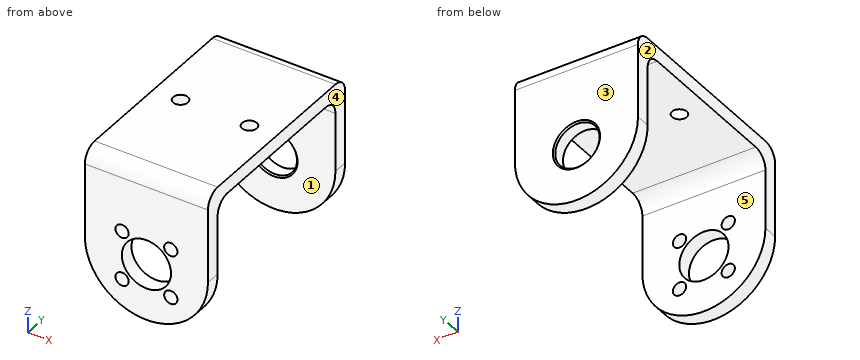
from build123d import *

# Parameters (mm, degrees)
BOSS_EXTRUDE3_DEPTH = 21.25
SHELL1_T            = -3
SKETCH6_R           = 4.5
CUT_EXTRUDE4_DEPTH  = 8.5
SKETCH8_R           = 1.347336496
CUT_EXTRUDE5_DEPTH  = 6
SKETCH9_R           = 1.5
CUT_EXTRUDE6_DEPTH  = 10
FILLET1_R           = 3
SKETCH11_R          = 5
CUT_EXTRUDE7_DEPTH  = 10
CHAMFER1_SIZE       = 0.3


with BuildPart() as part:
    # Sketch3 → Boss-Extrude3 (new, symmetric)
    with BuildSketch(Plane(origin=(0, 0, 0), x_dir=(1, 0, 0), z_dir=(0, 1, 0))):
        with BuildLine():
            Line((-12.5, 4), (12.5, 4))
            Line((12.5, 4), (12.5, 22))
            ThreePointArc((12.5, 22), (0, 34.5), (-12.5, 22))
            Line((-12.5, 22), (-12.5, 4))
        make_face()
    extrude(amount=BOSS_EXTRUDE3_DEPTH, both=True)

    # Shell1
    shell1_openings = [part.faces().sort_by_distance(p)[0] for p in [
        (0, 0, -34.5),
        (12.5, 0, -13),
        (-12.5, 0, -13),
    ]]
    offset(amount=SHELL1_T, openings=shell1_openings, kind=Kind.INTERSECTION)

    # Sketch6 → Cut-Extrude4 (cut)
    with BuildSketch(Plane(origin=(0, 21.25, 0), x_dir=(1, 0, 0), z_dir=(0, 1, 0))):
        with Locations(Location((0, 23, 0), (0, 0, 270))):
            Circle(SKETCH6_R)
    extrude(amount=-CUT_EXTRUDE4_DEPTH, mode=Mode.SUBTRACT)

    # Sketch8 → Cut-Extrude5 (cut)
    with BuildSketch(Plane(origin=(0, -21.25, 0), x_dir=(-1, 0, 0), z_dir=(0, -1, 0))):
        with Locations(Location((4.949747468, 18.050252532, 0), (0, 0, 90))):
            Circle(SKETCH8_R)
        with Locations(Location((-4.949747468, 18.050252532, 0), (0, 0, 90))):
            Circle(SKETCH8_R)
        with Locations(Location((-4.949747468, 27.949747468, 0), (0, 0, 90))):
            Circle(SKETCH8_R)
        with Locations(Location((4.949747468, 27.949747468, 0), (0, 0, 90))):
            Circle(SKETCH8_R)
    extrude(amount=-CUT_EXTRUDE5_DEPTH, mode=Mode.SUBTRACT)

    # Sketch9 → Cut-Extrude6 (cut)
    with BuildSketch(Plane(origin=(0, 0, -7), x_dir=(-1, 0, 0), z_dir=(0, 0, -1))):
        with Locations((-7, 0)):
            Circle(SKETCH9_R)
        with Locations((7, 0)):
            Circle(SKETCH9_R)
    extrude(amount=-CUT_EXTRUDE6_DEPTH, mode=Mode.SUBTRACT)

    # Fillet1
    fillet1_edges = [part.edges().sort_by_distance(p)[0] for p in [
        (0, -18.25, -7),
        (0, 18.25, -7),
        (0, -21.25, -4),
        (0, 21.25, -4),
    ]]
    fillet(fillet1_edges, radius=FILLET1_R)

    # Sketch11 → Cut-Extrude7 (cut)
    with BuildSketch(Plane(origin=(0, -18.25, 0), x_dir=(1, 0, 0), z_dir=(0, 1, 0))):
        with Locations(Location((0, 23, 0), (0, 0, 270))):
            Circle(SKETCH11_R)
    extrude(amount=-CUT_EXTRUDE7_DEPTH, mode=Mode.SUBTRACT)

    # Chamfer1
    chamfer1_edges = [part.edges().sort_by_distance(p)[0] for p in [
        (0, 18.25, -27.5),
        (0, 21.25, -27.5),
    ]]
    chamfer(chamfer1_edges, length=CHAMFER1_SIZE)


solid = part.part
Source: CAD feature listing. Evaluate the final solid. Frame: model axes, mm. Face numbers are marked on the shaded views. A direction names the side the tool comes from. Coordinates: 2 decimals unless noted, no trailing zeros. Loops run counter-clockwise (first coordinate to the right, second up) from the corner with the lowest first, then second, coordinate; pieces in that order, holes last. Notation, with made-up numbers: (34.25, 67.5) -> (72.25, 67.5) arc R31 ccw to (72.25, 99.5) -> close; hole circle Ø10 at (82.5, 87). An arc over 180 degrees is marked (long way). Answer in a Markdown table with one row per item. Add a question column.
Q1. Section D-D on z = -30.5. Return the cut outline in (x, y), and give its area (3 significant figures).
Q2. Pull-direction query (Y, two-part tool) for the marked faces 3, 4 and 5; classes: pulls with the +Y half, pulls with the -Y half, needs draft (parallel to the pull), parting line crosses it, or undercut.
Q3. Contact query for flat-ended pins moving along their axis: pin 1 Ø5 at (x, y) = (-7, 0) entering from -Z; pin 2 Ø2 at (x, z) = (-4.95, -27.95) entering from -Y. Output: stop coordinate, or through.
Q4. Section B-B on x = 0. Return the cut outline in (y, z).
Q5. Section A-A on y = 0. Return the cut outline in (x, z), and give its area (3 significant figures).
Q6. Section C-C on x = -7. Return the cut outline in (y, z).
Q7. Ray query, line 1 along Y through (x, z) = (-8, -29.5); line 2 along Z through (x, y) = (7.5, 9.5); line 3 along Y through (x, z) = (10.5, -8). Return the intervals inside material, ascending.
Q8. Reachability of the marked faces 1 and 2 from +Z, -Z, +X, -X, +Y, -Y: full face, straight path, thin tool, end or side. Return the list, or none.
Computed values:
| question | item | result |
|---|---|---|
| 1 | outline | (-9.17, -21.25) -> (9.17, -21.25) -> (9.17, -18.25) -> (-9.17, -18.25) -> close; (-9.17, 18.25) -> (9.17, 18.25) -> (9.17, 21.25) -> (-9.17, 21.25) -> close |
| 1 | area | 110 mm^2 |
| 2 | face 3 | pulls with the +Y half |
| 2 | face 4 | needs draft |
| 2 | face 5 | undercut |
| 3 | pin 1 | stops at z = -7 |
| 3 | pin 2 | stops at y = 18.25 |
| 4 | outline | (-21.25, -34.5) -> (-18.25, -34.5) -> (-18.25, -28) -> (-21.25, -28) -> close; (-21.25, -18) -> (-18.25, -18) -> (-18.25, -10) arc R3 cw to (-15.25, -7) -> (15.25, -7) arc R3 cw to (18.25, -10) -> (18.25, -18.2) -> (18.55, -18.5) -> (20.95, -18.5) -> (21.25, -18.2) -> (21.25, -7) arc R3 ccw to (18.25, -4) -> (-18.25, -4) arc R3 ccw to (-21.25, -7) -> close; (18.25, -34.5) -> (21.25, -34.5) -> (21.25, -27.8) -> (20.95, -27.5) -> (18.55, -27.5) -> (18.25, -27.8) -> close |
| 5 | outline | (-12.5, -7) -> (-8.5, -7) -> (-8.5, -4) -> (-12.5, -4) -> close; (-5.5, -7) -> (5.5, -7) -> (5.5, -4) -> (-5.5, -4) -> close; (8.5, -7) -> (12.5, -7) -> (12.5, -4) -> (8.5, -4) -> close |
| 5 | area | 57.0 mm^2 |
| 6 | outline | (-21.25, -32.36) -> (-18.25, -32.36) -> (-18.25, -10) arc R3 cw to (-15.25, -7) -> (-1.5, -7) -> (-1.5, -4) -> (-18.25, -4) arc R3 ccw to (-21.25, -7) -> close; (1.5, -7) -> (15.25, -7) arc R3 cw to (18.25, -10) -> (18.25, -32.36) -> (21.25, -32.36) -> (21.25, -7) arc R3 ccw to (18.25, -4) -> (1.5, -4) -> close |
| 7 | line 1 | y = -21.25 to -18.25, 18.25 to 21.25 |
| 7 | line 2 | z = -7 to -4 |
| 7 | line 3 | y = -21.25 to -17.49, 17.49 to 21.25 |
| 8 | face 1 | -Z, +X, -X |
| 8 | face 2 | +Z, -Z, -X, +Y, -Y |
